```python
from build123d import *

# Parameters (mm, degrees)
SKETCH1_R                      = 6.35
BOSS_EXTRUDE1_DEPTH            = 3.96875
F_3_16_0_1875_DIAMETER_HOLE1_D = 4.7625
CHAMFER1_SIZE                  = 0.254


with BuildPart() as part:
    # Sketch1 → Boss-Extrude1 (new body)
    with BuildSketch(Plane(origin=(0, 0, 0), x_dir=(1, 0, 0), z_dir=(0, 1, 0))):
        with Locations(Location((0, 0, 0), (0, 0, 270))):
            Circle(SKETCH1_R)
    extrude(amount=BOSS_EXTRUDE1_DEPTH)

    # 3/16 (0.1875) Diameter Hole1 (through all)
    with Locations(Plane(origin=(0, 3.96875, 0), x_dir=(1, 0, 0), z_dir=(0, 1, 0))):
        with Locations((0, 0)):
            Hole(F_3_16_0_1875_DIAMETER_HOLE1_D / 2)

    # Chamfer1
    chamfer1_edges = [part.edges().sort_by_distance(p)[0] for p in [
        (0, 0, -6.35),
        (0, 3.96875, -6.35),
        (2.38125, 3.96875, 0),
        (2.38125, 0, 0),
    ]]
    chamfer(chamfer1_edges, length=CHAMFER1_SIZE)


solid = part.part
```
Part model, mm, in its own coordinate system. Round coordinates to 2 decimals unless told otherwise and drop trailing zeros. Write each loop counter-clockwise with the first axis right and the second up, starting at its lowest first coordinate (ties: lowest second). Pieces come first, ordered by that corner, then holes. Notation, with made-up numbers: M 17,11.5 L 69,11.5 A19 ccw 69,42.5 Z; hole C 70,37 d8. An arc over 180 degrees is marked long. Answer as CSV lines item,"result". Start each with the question number.
1) Drill centre lines: L1, parallel to X at y = 1.65, z = 0; L2, parallel to X at y = 2.15, z = 1. Where is each one in solid material? Low to high.
2) Band-saw the part on A-A (z = 0). List the corners of the cut face in (x, y).
3) Band-saw the part on C-C (y = 3.3). List the corners of the cut face in (x, z), then the cut area to 3 significant figures.
4) Mould opens along X. For faces 1 (the face through (-1, 0, 3)), 2 (the face through (-3.86, 1.96, -5.04)), 3 (the face through (1.89, 1.96, 1.45)) say: +X half, -X half, draft (parallel to the pull), parting line (faces both ways), or undercut.
5) Band-saw the part on B-B (x = 0). List the corners of the cut face in (y, z), then the cut area to 3 significant figures.
6) Drop flat-ended pins along their axis: pin 1 (1 mm diameter, centred on x = -3.5, y = 1, fed in from -Z); pin 2 (1 mm diameter, centred on x = 1.5, y = 2, fed in from -Z); pin 3 (1 mm diameter, centred on y = 2, z = -2, fed in from +X); pin 4 (6 mm diameter, centred on x = -1, z = -1.5, fed in from +Y). Give the stop position or say it passes through.
Worked out:
1,L1,"-6.35 to -2.38, 2.38 to 6.35"
1,L2,"-6.27 to -2.16, 2.16 to 6.27"
2,outline,"M -6.35,0.25 L -6.1,0 L -2.64,0 L -2.38,0.25 L -2.38,3.71 L -2.64,3.97 L -6.1,3.97 L -6.35,3.71 Z; M 2.38,0.25 L 2.64,0 L 6.1,0 L 6.35,0.25 L 6.35,3.71 L 6.1,3.97 L 2.64,3.97 L 2.38,3.71 Z"
3,outline,"C 0,0 d12.7; hole C 0,0 d4.76"
3,area,"109 mm²"
4,face 1,"draft"
4,face 2,"parting line"
4,face 3,"undercut"
5,outline,"M 0,-6.1 L 0.25,-6.35 L 3.71,-6.35 L 3.97,-6.1 L 3.97,-2.64 L 3.71,-2.38 L 0.25,-2.38 L 0,-2.64 Z; M 0,2.64 L 0.25,2.38 L 3.71,2.38 L 3.97,2.64 L 3.97,6.1 L 3.71,6.35 L 0.25,6.35 L 0,6.1 Z"
5,area,"31.2 mm²"
6,pin 1,"z = -5.6"
6,pin 2,"z = -6.27"
6,pin 3,"x = 6.17"
6,pin 4,"y = 3.97"
